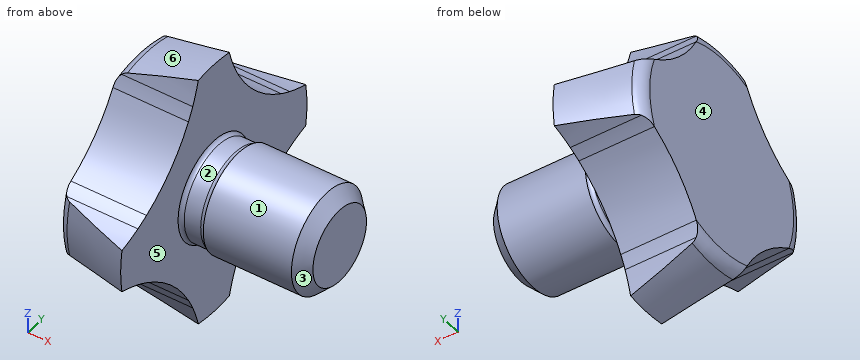
from build123d import *

# Parameters (mm, degrees)
F0_W     = 3.5
F0_H     = 2
F0_W_2   = 0.65359
F0_H_2   = 1.9
F3_DEPTH = 25


# Not quite as in the source:
# - ends of sketch curves that miss each other by under 0.0002 mm in the source are joined


with BuildPart() as f1:
    # F0 (on Front) → F1 (revolve)
    with BuildSketch(Plane.XZ):
        with BuildLine():
            ThreePointArc((6.2807068037, 4.5095537326), (6.0134401175, 4.3309714378), (5.910117, 4.026591))
            Line((5.910117, 4.026591), (5.910117, 0))
            Line((5.910117, 0), (8.910117, 0))
            Line((8.910117, 0), (8.910117, 1.999999965))
            Line((8.910117, 1.999999965), (8.910117, 5.214102))
            Line((8.910117, 5.214102), (6.2807068037, 4.5095537326))
        make_face()
        with BuildLine():
            Line((9.736912, 1.9), (9.736912, 0))
            Line((9.736912, 0), (9.910117, 0))
            Line((9.910117, 0), (9.910117, 2))
            ThreePointArc((9.9101170606, 1.999999965), (9.8369119825, 1.9267949091), (9.736912, 1.9))
        make_face()
        with Locations((11.660117, 1)):
            Rectangle(F0_W, F0_H)
        with Locations((9.410117, 0.95)):
            Rectangle(F0_W_2, F0_H_2)
        with BuildLine():
            Line((8.910117, 1.999999965), (8.910117, 0))
            Line((8.910117, 0), (9.083322, 0))
            Line((9.083322, 0), (9.083322, 1.9))
            ThreePointArc((9.083322, 1.9), (8.9833220175, 1.9267949091), (8.9101169394, 1.999999965))
        make_face()
        Polygon((13.410117, 2), (13.410117, 0), (13.910117, 0), (13.910117, 1.5), align=None)
    revolve(axis=Axis((10.414001145, 0, 0), (-1, 0, 0)))

    # F2 (on face) → F3 (cut)
    with BuildSketch(Plane(origin=(5.910117, 0, 0), x_dir=(0, -1, 0), z_dir=(-1, 0, 0))):
        with BuildLine():
            ThreePointArc((1.1816228772, -4.2490125583), (1.0079083628, -4.6889045584), (0.8693810599, -5.1411123543))
            ThreePointArc((0.8693810599, -5.1411123543), (3.686926882, -3.686926882), (5.1411123543, -0.8693810599))
            ThreePointArc((5.1411123543, -0.8693810599), (4.6889045584, -1.0079083628), (4.2490125583, -1.1816228772))
            ThreePointArc((4.2490125583, -1.1816228772), (4.0057430921, -1.2955299839), (3.7678156951, -1.420211241))
            ThreePointArc((3.7678156951, -1.420211241), (2.8472298012, -2.8472298012), (1.420211241, -3.7678156951))
            ThreePointArc((1.420211241, -3.7678156951), (1.2955299839, -4.0057430921), (1.1816228772, -4.2490125583))
        make_face()
        with BuildLine():
            ThreePointArc((-5.1411123543, -0.8693810599), (-3.686926882, -3.686926882), (-0.8693810599, -5.1411123543))
            ThreePointArc((-0.8693810599, -5.1411123543), (-1.0079083664, -4.6889048876), (-1.1816228201, -4.2490132008))
            ThreePointArc((-1.1816228201, -4.2490132008), (-1.2955301515, -4.0057433246), (-1.4202116652, -3.7678155352))
            ThreePointArc((-1.4202116652, -3.7678155352), (-2.8472298012, -2.8472298012), (-3.7678155352, -1.4202116652))
            ThreePointArc((-3.7678155352, -1.4202116652), (-4.0057429748, -1.2955303249), (-4.2490124865, -1.1816231353))
            ThreePointArc((-4.2490124865, -1.1816231353), (-4.6889045191, -1.0079084953), (-5.1411123543, -0.8693810599))
        make_face()
        with BuildLine():
            ThreePointArc((4.2490125583, 1.1816228772), (4.6889045584, 1.0079083628), (5.1411123543, 0.8693810599))
            ThreePointArc((5.1411123543, 0.8693810599), (3.686926882, 3.686926882), (0.8693810599, 5.1411123543))
            ThreePointArc((0.8693810599, 5.1411123543), (1.0079083628, 4.6889045584), (1.1816228772, 4.2490125583))
            ThreePointArc((1.1816228772, 4.2490125583), (1.2955299839, 4.0057430921), (1.420211241, 3.7678156951))
            ThreePointArc((1.420211241, 3.7678156951), (2.8472298012, 2.8472298012), (3.7678156951, 1.420211241))
            ThreePointArc((3.7678156951, 1.420211241), (4.0057430921, 1.2955299839), (4.2490125583, 1.1816228772))
        make_face()
        with BuildLine():
            ThreePointArc((3.7678156951, -1.420211241), (2.4284046412, -2.4284046412), (1.420211241, -3.7678156951))
            ThreePointArc((1.420211241, -3.7678156951), (2.8472298012, -2.8472298012), (3.7678156951, -1.420211241))
        make_face()
        with BuildLine():
            ThreePointArc((-0.8693810599, 5.1411123543), (-3.686926882, 3.686926882), (-5.1411123543, 0.8693810599))
            ThreePointArc((-5.1411123543, 0.8693810599), (-4.6889043312, 1.0079080153), (-4.2490121021, 1.1816222641))
            ThreePointArc((-4.2490121021, 1.1816222641), (-4.0057431642, 1.295528931), (-3.7678162701, 1.4202097156))
            ThreePointArc((-3.7678162701, 1.4202097156), (-2.8472298012, 2.8472298012), (-1.4202097156, 3.7678162701))
            ThreePointArc((-1.4202097156, 3.7678162701), (-1.2955287576, 4.0057435139), (-1.181621949, 4.2490128164))
            ThreePointArc((-1.181621949, 4.2490128164), (-1.0079078864, 4.6889046997), (-0.8693810599, 5.1411123543))
        make_face()
        with BuildLine():
            ThreePointArc((-3.7678155352, -1.4202116652), (-2.8472298012, -2.8472298012), (-1.4202116652, -3.7678155352))
            ThreePointArc((-1.4202116652, -3.7678155352), (-2.4284049327, -2.4284049327), (-3.7678155352, -1.4202116652))
        make_face()
        with BuildLine():
            ThreePointArc((1.420211241, 3.7678156951), (2.4284046412, 2.4284046412), (3.7678156951, 1.420211241))
            ThreePointArc((3.7678156951, 1.420211241), (2.8472298012, 2.8472298012), (1.420211241, 3.7678156951))
        make_face()
        with BuildLine():
            ThreePointArc((-1.4202097156, 3.7678162701), (-2.8472298012, 2.8472298012), (-3.7678162701, 1.4202097156))
            ThreePointArc((-3.7678162701, 1.4202097156), (-2.428403593, 2.428403593), (-1.4202097156, 3.7678162701))
        make_face()
    extrude(amount=-F3_DEPTH, mode=Mode.SUBTRACT)


solid = f1.part
For this review, take the finished solid that the model builds, in its own axes (mm). Face numbers are marked on the shaded views. A direction names the side the tool comes from. Round coordinates to 2 decimals unless told otherwise and drop trailing zeros. Loops run counter-clockwise (first coordinate to the right, second up) from the corner with the lowest first, then second, coordinate; pieces in that order, holes last. Notation, with made-up numbers: (61, 56.25) - (117, 56.25) arc R21 cw to (117, 75.25) - close; hole circle Ø8 at (-13.5, -34.75). An arc over 180 degrees is marked (long way). One line per question, with ' | ' between items.
Q1. Take a section at B-B (x = 6.75). Give the boundary of the cut face in (y, z).
Taken from the geometry:
outline: (-4.51, -1.07) arc R6 cw to (-1.07, -4.51) arc R4.64 ccw to (1.07, -4.51) arc R6 cw to (4.51, -1.07) arc R4.64 ccw to (4.51, 1.07) arc R6 cw to (1.07, 4.51) arc R4.64 ccw to (-1.07, 4.51) arc R6 cw to (-4.51, 1.07) arc R4.64 ccw to start
Q2. For line 1 along X through (y, z) = (1.75, 2.25); line 2 along Z through (x, y) = (9, -0.25); line 3 along Y through (x, z) = (11, 0), list the stretches that pass through material, from the lowest coordinate up. Write a range as [from, to].
Taken from the geometry:
line 1: x = [5.91, 8.91] | line 2: z = [-1.9, 1.9] | line 3: y = [-2, 2]
Q3. Take a section at D-D (x = 11). Give the boundary of the cut face in (y, z).
Taken from the geometry:
outline: circle Ø4 at (0, 0)
Q4. Tool access review of the marked faces 5 and 6: name each direction out of +Z, -Z, +X, -X, +Y, -Y from which nothing blocks a thin tool from reaching the whole face with its end or side.
Taken from the geometry:
face 5: +X | face 6: +Z, -X
Q5. Take a section at A-A (y = 0). Give the boundary of the cut face in (x, z).
Taken from the geometry:
outline: (5.91, -4.03) arc R0.5 ccw to (6.28, -4.51) - (8.91, -5.21) - (8.91, -2) arc R0.2 cw to (9.08, -1.9) - (9.74, -1.9) arc R0.2 cw to (9.91, -2) - (13.41, -2) - (13.91, -1.5) - (13.91, 1.5) - (13.41, 2) - (9.91, 2) arc R0.2 cw to (9.74, 1.9) - (9.08, 1.9) arc R0.2 cw to (8.91, 2) - (8.91, 5.21) - (6.28, 4.51) arc R0.5 ccw to (5.91, 4.03) - close
Q6. The part is to be moulded in two halves that separate along X. For the marked faces 1, 2, 3 and 4, say which applies: released by +X, released by -X, zero draft, split by the parting line, or undercut.
Taken from the geometry:
face 1: zero draft | face 2: undercut | face 3: released by +X | face 4: released by -X
Q7. For pin 1 (1 mm diameter, centred on x = 12, z = 3, fed in from -Y); pin 2 (1 mm diameter, centred on x = 7, y = -2.5, fed in from +Z), all flat-tipped, find the tip position at first contact; note any pin that passes through.
Taken from the geometry:
pin 1: passes through | pin 2: stops at z = 2.91
